Could you check a few things on this model? Use its own coordinates, in mm. A direction names the side the tool comes from. Round coordinates to 2 decimals unless told otherwise and drop trailing zeros. Write each loop counter-clockwise with the first axis right and the second up, starting at its lowest first coordinate (ties: lowest second). Pieces come first, ordered by that corner, then holes. Notation, with made-up numbers: (85, -14.75) -> (132, -14.75) arc R20 cw to (132, -1.75) -> close; hole circle Ø7 at (69, 28). An arc over 180 degrees is marked (long way). Answer in a Markdown table with one row per item.
from build123d import *

# Parameters (mm, degrees)
BOSS_EXTRUDE2_DEPTH = 30
SKETCH2_R           = 1.5
CUT_EXTRUDE1_DEPTH  = 66
SKETCH3_R           = 6.25
SKETCH3_R_2         = 1.5
CUT_EXTRUDE2_DEPTH  = 10
FILLET1_R           = 2


with BuildPart() as part:
    # Sketch1 → Boss-Extrude2 (new body)
    with BuildSketch(Plane(origin=(0, 0, 0), x_dir=(1, 0, 0), z_dir=(0, 1, 0))):
        Polygon((0, -38.328427125), (23.171572875, -38.328427125), (30.5, -31), (30.5, 0), (32.5, 0), (32.5, -31.828427125), (24, -40.328427125), (0, -40.328427125), align=None)
    boss_extrude2 = extrude(amount=BOSS_EXTRUDE2_DEPTH)

    # Mirror1: Boss-Extrude2 across plane
    add(boss_extrude2.mirror(Plane(origin=(0, 0, 0), x_dir=(0, 0, 1), z_dir=(1, 0, 0))))

    # Sketch2 → Cut-Extrude1 (cut, through all)
    with BuildSketch(Plane(origin=(32.5, 0, 0), x_dir=(0, 0, -1), z_dir=(1, 0, 0))):
        with Locations((-17, 15)):
            Circle(SKETCH2_R)
        with Locations((-5, 3)):
            Circle(SKETCH2_R)
        with Locations((-13.5, 6.5)):
            Circle(SKETCH2_R)
        with Locations((-13.5, 23.5)):
            Circle(SKETCH2_R)
        with Locations((-5, 27)):
            Circle(SKETCH2_R)
        with BuildLine():
            Line((-4.75, 21.25), (0, 21.25))
            Line((0, 21.25), (0, 8.75))
            Line((0, 8.75), (-4.75, 8.75))
            ThreePointArc((-4.75, 8.75), (-11, 15), (-4.75, 21.25))
        make_face()
    extrude(amount=-CUT_EXTRUDE1_DEPTH, mode=Mode.SUBTRACT)

    # Sketch3 → Cut-Extrude2 (cut)
    with BuildSketch(Plane.XY.offset(40.328427125)):
        with Locations((0, 15)):
            Circle(SKETCH3_R)
        with Locations((8.470537173, 6.5)):
            Circle(SKETCH3_R_2)
        with Locations((8.470537173, 23.5)):
            Circle(SKETCH3_R_2)
        with Locations((19.970537173, 5)):
            Circle(SKETCH3_R_2)
        with Locations((19.970537173, 25)):
            Circle(SKETCH3_R_2)
        with Locations((-19.970537173, 5)):
            Circle(SKETCH3_R_2)
        with Locations((-8.470537173, 6.5)):
            Circle(SKETCH3_R_2)
        with Locations((-19.970537173, 25)):
            Circle(SKETCH3_R_2)
        with Locations((-8.470537173, 23.5)):
            Circle(SKETCH3_R_2)
    extrude(amount=-CUT_EXTRUDE2_DEPTH, mode=Mode.SUBTRACT)

    # Fillet1
    fillet1_edges = [part.edges().sort_by_distance(p)[0] for p in [
        (31.5, 0, 0),
        (32.5, 15, 31.828427125),
        (24, 15, 40.328427125),
        (23.171572875, 15, 38.328427125),
        (30.5, 15, 31),
        (-31.5, 30, 0),
        (-32.5, 15, 31.828427125),
        (-24, 15, 40.328427125),
        (-23.171572875, 15, 38.328427125),
        (-30.5, 15, 31),
        (-31.5, 0, 0),
        (31.5, 30, 0),
        (31.5, 21.25, 0),
        (31.5, 8.75, 0),
        (-31.5, 21.25, 0),
        (-31.5, 8.75, 0),
    ]]
    fillet(fillet1_edges, radius=FILLET1_R)


solid = part.part
1) Imagine slicing it at D-D, the plane x = 9. Please give me the cut outline in (y, z).
Findings:
| item | result |
|---|---|
| outline | (0, 38.33) -> (5.1, 38.33) -> (5.1, 40.33) -> (0, 40.33) -> close; (7.9, 38.33) -> (22.1, 38.33) -> (22.1, 40.33) -> (7.9, 40.33) -> close; (24.9, 38.33) -> (30, 38.33) -> (30, 40.33) -> (24.9, 40.33) -> close |
2) Imagine slicing it at C-C, the plane z = 28.5. Please give me the cut outline in (x, y), plus the area to 3 significant figures.
Findings:
| item | result |
|---|---|
| outline | (-32.5, 0) -> (-30.5, 0) -> (-30.5, 30) -> (-32.5, 30) -> close; (30.5, 0) -> (32.5, 0) -> (32.5, 30) -> (30.5, 30) -> close |
| area | 120 mm^2 |
3) Please list where these lines run through material, in increasing order: line 1 (Y direction, x = 31.1, z = 13.5); line 2 (Y direction, x = 31.35, z = 5) (3 decimals); line 3 (X direction, y = 27.25, z = 25).
Findings:
| item | result |
|---|---|
| line 1 | y = 0 to 5, 8 to 22, 25 to 30 |
| line 2 | y = 0 to 1.5, 4.5 to 8.755, 21.245 to 25.5, 28.5 to 30 |
| line 3 | x = -32.5 to -30.5, 30.5 to 32.5 |
4) Imagine slicing it at A-A, the plane z = 13.5. Please give me the cut outline in (x, y), plus the area to 3 significant figures.
Findings:
| item | result |
|---|---|
| outline | (-32.5, 0) -> (-30.5, 0) -> (-30.5, 5) -> (-32.5, 5) -> close; (-32.5, 8) -> (-30.5, 8) -> (-30.5, 22) -> (-32.5, 22) -> close; (-32.5, 25) -> (-30.5, 25) -> (-30.5, 30) -> (-32.5, 30) -> close; (30.5, 0) -> (32.5, 0) -> (32.5, 5) -> (30.5, 5) -> close; (30.5, 8) -> (32.5, 8) -> (32.5, 22) -> (30.5, 22) -> close; (30.5, 25) -> (32.5, 25) -> (32.5, 30) -> (30.5, 30) -> close |
| area | 96.0 mm^2 |
5) For pin 1 (15 mm diameter, centred on x = -7.5, y = 20, fed in from -Z), with a flat end and sliding along its axis, tell me the tip position at first contact or that it passes through.
Findings:
| item | result |
|---|---|
| pin 1 | stops at z = 38.33 |
6) Thinking about a two-plate mould opening in Y: for faces 4 (the face through (-26.8, 14.8, 34.7)), 5 (the face through (-31.51, 21.85, 0.57)), 6 (the face through (0, 0, 40)), which applies, +Y half, -Y half, draft (parallel to the pull), parting line (faces both ways), or undercut?
Findings:
| item | result |
|---|---|
| face 4 | draft |
| face 5 | undercut |
| face 6 | -Y half |
7) Imagine slicing it at B-B, the plane y = 15. Count the separate pieces of the cut face and the enclosed holes in it, plus the area to 3 significant figures.
Findings:
| item | result |
|---|---|
| separate pieces | 4 |
| enclosed holes | 0 |
| area | 184 mm^2 |
8) For faces 1 (the face through (32, 21.25, 3)), 2 (the face through (-31.5, 5.6, 14.7)), 3 (the face through (-23.1, 15.21, 38.18)), which set-ups out of +Z, -Z, +X, -X, +Y, -Y let a thin tool reach every point of the face, with its end or its side?
Findings:
| item | result |
|---|---|
| face 1 | -Z, +X, -X |
| face 2 | +X, -X |
| face 3 | -Z, +Y, -Y |
